Could you check a few things on this model? Use its own coordinates, in mm. Round coordinates to 2 decimals unless told otherwise and drop trailing zeros. Write each loop counter-clockwise with the first axis right and the second up, starting at its lowest first coordinate (ties: lowest second). Pieces come first, ordered by that corner, then holes. Notation, with made-up numbers: M 46.5,-3 L 96.5,-3 A18 cw 96.5,19 Z; hole C 9,19 d7. An arc over 180 degrees is marked long. One line per item, written item: value. Start each with the question number.
(1) I want a section at D-D on x = 120. Please give me the cut outline in (y, z).
(2) I'm going to push flat-ended pins straight in: pin 1 Ø10 at (x, y) = (10, -43) entering from +Z; pin 2 Ø12 at (x, y) = (43.5, -12.5) entering from +Z; pin 3 Ø5 at (x, z) = (82.5, -23.5) entering from -Y. Where does each tip first touch, or does it pass through?
(3) Thinking about a two-plate mould opening in Z: for faces 1 (the face through (120, -75, -18)), 2 (the face through (68.616, -22.185, 36.506)), 3 (the face through (-2.76, -4.76, -12.44)), which applies, released by +Z, released by -Z, zero draft, split by the parting line, or undercut?
(4) If I drill on L1, parallel to Z at x = 0, y = -46.5; L2, parallel to X at y = -35.5, z = -1.5; L3, parallel to Y at x = 106.5, z = 27, over which ranges is the centre line in solid material (lowest first)?
(5) I want a section at A-A on x = 0. Please give me the cut outline in (y, z).
(6) I want a section at C-C on z = -10.5. Count the separate pieces of the cut face and the enclosed holes in it, and give its area (3 significant figures).
(7) I want a section at B-B on y = -15. Please give me the cut outline in (x, z).
```python
from build123d import *

# Parameters (mm, degrees)
F0_R     = 12.5
F1_DEPTH = 45
F2_DEPTH = 75
F3_SIZE  = 5
F4_SIZE  = 5
F5_DEPTH = 15


with BuildPart() as f1:
    # F0 (on Front) → F1 (new body)
    with BuildSketch(Plane.XZ):
        with BuildLine():
            ThreePointArc((10.416667, -48.902894), (38.864079, -31.457643), (50, 0))
            ThreePointArc((50, 0), (38.864079, 31.457643), (10.416667, 48.902894))
            ThreePointArc((10.416667, 48.902894), (-50, 0), (10.416667, -48.902894))
        make_face()
        Circle(F0_R, mode=Mode.SUBTRACT)
        with BuildLine():
            ThreePointArc((10.416667, 48.902894), (38.864079, 31.457643), (50, 0))
            ThreePointArc((50, 0), (38.864079, -31.457643), (10.416667, -48.902894))
            Line((10.416667, -48.902894), (125.208333, -24.451447))
            ThreePointArc((125.208333, -24.451447), (95, 0), (125.208333, 24.451447))
            Line((125.208333, 24.451447), (10.416667, 48.902894))
        make_face()
        with BuildLine():
            ThreePointArc((145, 0), (139.43204, 15.728822), (125.208333, 24.451447))
            ThreePointArc((125.208333, 24.451447), (95, 0), (125.208333, -24.451447))
            ThreePointArc((125.208333, -24.451447), (139.43204, -15.728822), (145, 0))
        make_face()
        with Locations((120, 0)):
            Circle(F0_R, mode=Mode.SUBTRACT)
    extrude(amount=F1_DEPTH)

    # F0 (on Front) → F2 (join)
    with BuildSketch(Plane.XZ):
        with BuildLine():
            ThreePointArc((10.416667, -48.902894), (38.864079, -31.457643), (50, 0))
            ThreePointArc((50, 0), (38.864079, 31.457643), (10.416667, 48.902894))
            ThreePointArc((10.416667, 48.902894), (-50, 0), (10.416667, -48.902894))
        make_face()
        Circle(F0_R, mode=Mode.SUBTRACT)
        with BuildLine():
            ThreePointArc((145, 0), (139.43204, 15.728822), (125.208333, 24.451447))
            ThreePointArc((125.208333, 24.451447), (95, 0), (125.208333, -24.451447))
            ThreePointArc((125.208333, -24.451447), (139.43204, -15.728822), (145, 0))
        make_face()
        with Locations((120, 0)):
            Circle(F0_R, mode=Mode.SUBTRACT)
    extrude(amount=F2_DEPTH)

    # F3
    f3_edges = [f1.edges().sort_by_distance(p)[0] for p in [
        (-10.416667, -75, 48.902894),
        (-12.5, -75, 0),
        (114.791667, -75, 24.451447),
        (107.5, -75, 0),
    ]]
    chamfer(f3_edges, length=F3_SIZE)

    # F4
    f4_edges = [f1.edges().sort_by_distance(p)[0] for p in [
        (107.5, 0, 0),
        (-12.5, 0, 0),
    ]]
    chamfer(f4_edges, length=F4_SIZE)

    # F0 (on Front) → F5 (join)
    with BuildSketch(Plane.XZ):
        with BuildLine():
            ThreePointArc((10.416667, 48.902894), (38.864079, 31.457643), (50, 0))
            ThreePointArc((50, 0), (38.864079, -31.457643), (10.416667, -48.902894))
            Line((10.416667, -48.902894), (125.208333, -24.451447))
            ThreePointArc((125.208333, -24.451447), (95, 0), (125.208333, 24.451447))
            Line((125.208333, 24.451447), (10.416667, 48.902894))
        make_face()
    extrude(amount=F5_DEPTH)


solid = f1.part
```
Found:
1. outline: M -75,-20 L -70,-25 L -45,-25 L -45,-25.56 L 0,-25.56 L 0,-17.5 L -5,-12.5 L -70,-12.5 L -75,-17.5 Z; M -75,17.5 L -70,12.5 L -5,12.5 L 0,17.5 L 0,25.56 L -45,25.56 L -45,25 L -70,25 L -75,20 Z
2. pin 1: stops at z = 49.75
2. pin 2: stops at z = 43.13
2. pin 3: stops at y = -45
3. face 1: zero draft
3. face 2: released by +Z
3. face 3: undercut
4. L1: z = -50 to -12.5, 12.5 to 50
4. L2: x = -49.98 to -12.41, 12.41 to 107.59, 132.41 to 144.95
4. L3: y = -45 to 0
5. outline: M -75,-45 L -70,-50 L 0,-50 L 0,-17.5 L -5,-12.5 L -70,-12.5 L -75,-17.5 Z; M -75,17.5 L -70,12.5 L -5,12.5 L 0,17.5 L 0,50 L -70,50 L -75,45 Z
6. separate pieces: 3
6. enclosed holes: 0
6. area: 10,700 mm²
7. outline: M 10.42,-48.9 L 125.21,-24.45 A25 ccw 145,0 A25 ccw 125.21,24.45 L 10.42,48.9 A50 ccw long Z; hole C 0,0 d25; hole C 120,0 d25
